The figure shows three views and two pictorial views of one solid part (mm, origin at its lowest corner). Answer the questions. A direction names the side the tool comes from. Round coordinates to 2 decimals unless told otherwise and drop trailing zeros. Order: outer loops, then holes, each group sorted by start corner. A loop starts at its lowest first (then second) coordinate and runs counter-clockwise, first axis right, second up. Notation, with made-up numbers: (65, 41) - (84, 41) arc R28 cw to (84, 71) - close; hole circle Ø5 at (0.5, 37). An arc over 180 degrees is marked (long way). Use CSV: the item, a comma, the result in double quotes. Start each with the question number.
Item 1: Find section A-A, the plane x = 5. Give the vertices of the cut face in (y, z).
Item 2: Find section C-C, the plane z = 1.8. Give the vertices of the cut face in (x, y), plus the area to 3 significant figures.
Item 3: Straight lines are drawn through the part: line 1 along Y through (x, z) = (13.75, 1.4); line 2 along X through (y, z) = (17, 0.8); line 3 along Y through (x, z) = (11.25, 0.85). For each, find the intervals that lie inside material, in ascending order. Write a range as [from, to].
Item 4: Find section D-D, the plane x = 20. Give the vertices of the cut face in (y, z), plus the area to 3 significant figures.
Item 5: Find section B-B, the plane y = 17.25. Give the vertices of the cut face in (x, z), plus the area to 3 significant figures.
Item 6: Flat-ended cylindrical pins translate along their axes: P1, Ø0.9, axis at y = 16, z = 1.5, coming from the -X side; P2, Ø1, axis at y = 20.5, z = 2, coming from the -X side; P3, Ø1.2, axis at x = 21, z = 1, coming from the +Y side. Find the tip coordinate at first contact, or state that the pin passes through.
Item 7: Determine the mould class of the marked faces 1, 2 and 3 for opening direction Y: +Y half, -Y half, draft (parallel to the pull), parting line (faces both ways), or undercut.
Item 8: For the marked faces 4, 5 and 6, determine the directions among +Z, -Z, +X, -X, +Y, -Y from which every point of the face is accessible in a straight line to the end or side of a thin tool.
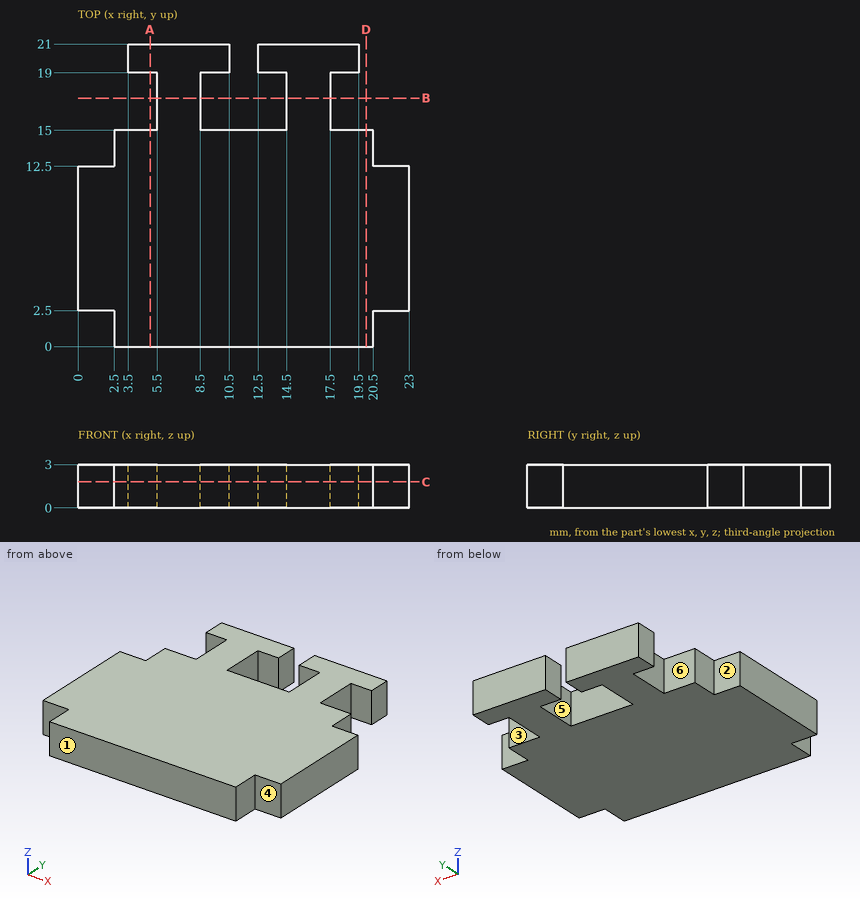
Worked out:
1,outline,"(0, 0) - (15, 0) - (15, 3) - (0, 3) - close; (19, 0) - (21, 0) - (21, 3) - (19, 3) - close"
2,outline,"(0, 2.5) - (2.5, 2.5) - (2.5, 0) - (20.5, 0) - (20.5, 2.5) - (23, 2.5) - (23, 12.5) - (20.5, 12.5) - (20.5, 15) - (17.5, 15) - (17.5, 19) - (19.5, 19) - (19.5, 21) - (12.5, 21) - (12.5, 19) - (14.5, 19) - (14.5, 15) - (8.5, 15) - (8.5, 19) - (10.5, 19) - (10.5, 21) - (3.5, 21) - (3.5, 19) - (5.5, 19) - (5.5, 15) - (2.5, 15) - (2.5, 12.5) - (0, 12.5) - close"
2,area,"372 mm²"
3,line 1,"y = [0, 15], [19, 21]"
3,line 2,"x = [5.5, 8.5], [14.5, 17.5]"
3,line 3,"y = [0, 15]"
4,outline,"(0, 0) - (15, 0) - (15, 3) - (0, 3) - close"
4,area,"45.0 mm²"
5,outline,"(5.5, 0) - (8.5, 0) - (8.5, 3) - (5.5, 3) - close; (14.5, 0) - (17.5, 0) - (17.5, 3) - (14.5, 3) - close"
5,area,"18.0 mm²"
6,P1,"stops at x = 5.5"
6,P2,"stops at x = 3.5"
6,P3,"stops at y = 15"
7,face 1,"-Y half"
7,face 2,"+Y half"
7,face 3,"undercut"
8,face 4,"+Z, -Z, +X, -Y"
8,face 5,"+Z, -Z"
8,face 6,"+Z, -Z, -X"
